Work out the finished part from the listing and answer in its coordinate system (mm). Give positions to 0.01 mm unless a question says otherwise; leave off trailing zeros. Write each loop counter-clockwise with the first axis right and the second up, starting at its lowest first coordinate (ties: lowest second). Pieces come first, ordered by that corner, then holes.
1) Straight lines are drawn through the part: probe 1 along X at (y, z) = (1.45, -35); probe 2 along Z at (x, y) = (-9, 1.9); probe 3 along Z at (x, y) = (-11.5, 2.3). For each, find the intervals that lie inside material, in ascending order.
2) Find section D-D (z = -41). Determine the outline of the cut face in (x, y), plus the area to 3 significant figures.
3) Find section B-B (y = 1.05). Determine the outline of the cut face in (x, z).
4) Find section A-A (x = -2). Determine the outline of the cut face in (y, z).
5) Find section C-C (x = -10). Determine the outline of the cut face in (y, z).
6) Given pin 1 Ø3.5 at (x, z) = (-2, 41) entering from +Y, flat-ended and moving along its own axis, determine where the tip first touches the part or whether it passes through.
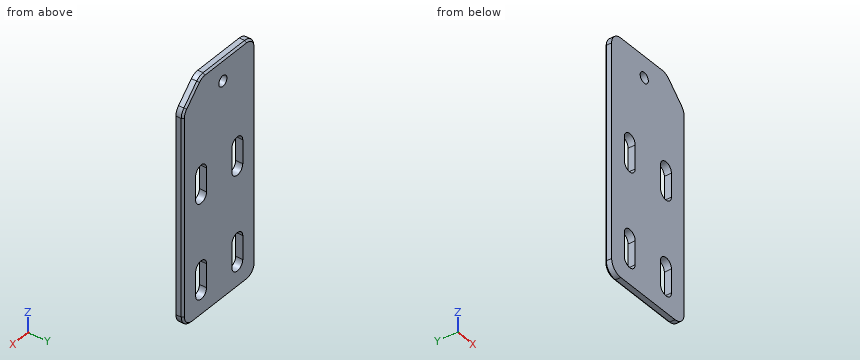
Autodesk Inventor part; units mm, degrees
ref_plane "YZ Plane" through (0, 0, 0) normal (1, 0, 0) x (0, 1, 0)
ref_plane "XZ Plane" through (0, 0, 0) normal (0, 1, 0) x (-1, 0, 0)
ref_plane "XY Plane" through (0, 0, 0) normal (0, 0, 1) x (1, 0, 0)
sketch "Sketch1" plane through (0, 0, 0) normal (0, 1, 0) x (-1, 0, 0)
  line L0 (-20, 50) -> (20, 50)
  line L1 (20, 50) -> (20, -50)
  line L2 (20, -50) -> (-20, -50)
  line L3 (-20, -50) -> (-20, 50)
  line L4 (-20, 50) -> (20, -50) construction
  line L5 (20, 50) -> (-20, -50) construction
  point P0 (0, 0)
  dimension "d0" = 100
  dimension "d1" = 40
extrude "Extrusion1" add sketch "Sketch1" along normal blind 3
sketch "Sketch2" plane through (0, 3, 0) normal (0, 1, 0) x (1, 0, 0)
  line L0 (-10, -10) -> (-10, 0) construction
  line L1 (-7, -10) -> (-7, 0)
  line L2 (-13, 0) -> (-13, -10)
  arc A0 (-13, -10) -> (-7, -10) centre (-10, -10) ccw
  arc A1 (-7, 0) -> (-13, 0) centre (-10, 0) ccw
  line L3 (-32, 15) -> (32, 15) construction
  line L4 (20, 50) -> (-20, 50)
  line L5 (0, 82) -> (0, -72)
  line L6 (-10, 40) -> (-10, 30) construction
  line L7 (-7, 40) -> (-7, 30)
  line L8 (-13, 30) -> (-13, 40)
  arc A2 (-7, 40) -> (-13, 40) centre (-10, 40) ccw
  arc A3 (-13, 30) -> (-7, 30) centre (-10, 30) ccw
  line L9 (10, -10) -> (10, 0) construction
  line L10 (7, -10) -> (7, 0)
  line L11 (13, 0) -> (13, -10)
  arc A4 (7, -10) -> (13, -10) centre (10, -10) ccw
  arc A5 (13, 0) -> (7, 0) centre (10, 0) ccw
  line L12 (10, 40) -> (10, 30) construction
  line L13 (7, 40) -> (7, 30)
  line L14 (13, 30) -> (13, 40)
  arc A6 (13, 40) -> (7, 40) centre (10, 40) ccw
  arc A7 (7, 30) -> (13, 30) centre (10, 30) ccw
  point P0 (0, 0)
  point P1 (-10, -5)
  point P2 (-10, 35)
  point P3 (10, -5)
  point P4 (10, 35)
  dimension "d4" = 3
  dimension "d5" = 10
  dimension "d6" = 20
  dimension "d7" = 35
  dimension "d8" = 10
  dimension "d24" = 40
sketch "Sketch3" plane through (0, 3, 0) normal (0, 1, 0) x (1, 0, 0)
  circle A0 centre (-2, -41) radius 2.25
  line L0 (-20, -50) -> (20, -50)
  line L1 (20, -50) -> (20, 50)
  line L2 (-20, 50) -> (-20, -50)
  point P0 (0, 0)
  dimension "d9" = 4.5
  dimension "d10" = 9
  dimension "d16" = 18
extrude "Extrusion2" cut sketch "Sketch3" against normal blind 3
extrude "Extrusion3" cut sketch "Sketch2" against normal blind 3
chamfer "Chamfer3" distance 10 angle 45 1 edges at (20, 1.5, 50)
fillet "Fillet2" radius 5 5 edges at (20, 1.5, 40) (10, 1.5, 50) (20, 1.5, -50) (-20, 1.5, -50) (-20, 1.5, 50)
chamfer "Chamfer4" distance 0.75 angle 45 10 edges at (20, 3, -3.5355) (18.5355, 3, -48.5355) (0, 3, -50) (-18.5355, 3, -48.5355) (-20, 3, 0) (-18.5355, 3, 48.5355) (-3.5355, 3, 50) (9.8423, 3, 49.6194) (15, 3, 45) (19.6194, 3, 39.8423)
properties part number "Middle"
Results:
1. probe 1: x = -20 to -13, -7 to 7, 13 to 20
1. probe 2: z = -50 to -42.83, -27.17 to -2.83, 12.83 to 50
1. probe 3: z = -49.95 to -42.6, -27.4 to -2.6, 12.6 to 49.95
2. outline: (-20, 0) - (-12.83, 0) - (-12.83, 3) - (-19.25, 3) - (-20, 2.25) - close; (-7.17, 0) - (7.17, 0) - (7.17, 3) - (-7.17, 3) - close; (12.83, 0) - (20, 0) - (20, 2.25) - (19.25, 3) - (12.83, 3) - close
2. area: 85.5 mm2
3. outline: (-20, -45) arc R5 ccw to (-15, -50) - (15, -50) arc R5 ccw to (20, -45) - (20, 37.93) arc R5 ccw to (18.54, 41.46) - (11.46, 48.54) arc R5 ccw to (7.93, 50) - (-15, 50) arc R5 ccw to (-20, 45) - close; hole (-13, -40) arc R3 ccw to (-7, -40) - (-7, -30) arc R3 ccw to (-13, -30) - close; hole (-13, 0) arc R3 ccw to (-7, 0) - (-7, 10) arc R3 ccw to (-13, 10) - close; hole circle Ø4.5 at (-2, 41); hole (7, -40) arc R3 ccw to (13, -40) - (13, -30) arc R3 ccw to (7, -30) - close; hole (7, 0) arc R3 ccw to (13, 0) - (13, 10) arc R3 ccw to (7, 10) - close
4. outline: (0, -50) - (2.25, -50) - (3, -49.25) - (3, 38.75) - (0, 38.75) - close; (0, 43.25) - (3, 43.25) - (3, 49.25) - (2.25, 50) - (0, 50) - close
5. outline: (0, -50) - (2.25, -50) - (3, -49.25) - (3, -43) - (0, -43) - close; (0, -27) - (3, -27) - (3, -3) - (0, -3) - close; (0, 13) - (3, 13) - (3, 49.25) - (2.25, 50) - (0, 50) - close
6. pin 1: passes through
